```python
from build123d import *

# Parameters (mm, degrees)
F0_R     = 3.175
F0_W     = 5.842
F0_H     = 12.7
F1_DEPTH = 25.4


with BuildPart() as f1:
    # F0 (on Front) → F1 (new body)
    with BuildSketch(Plane.XZ):
        Polygon((5.842, 12.7), (5.842, 0), (66.294, 0), (66.294, 12.7), (56.134, 12.7), (56.134, 10.16), (10.16, 10.16), (10.16, 12.7), align=None)
        with BuildLine():
            ThreePointArc((-8.1826630726, -5.5069827884), (-3.1957909266, -4.5493385486), (-0.9398, 0))
            ThreePointArc((-0.9398, 0), (-4.5919612295, 5.3297205562), (-10.8806298187, 3.8475430269))
            ThreePointArc((-10.8806298187, 3.8475430269), (-12.1459778134, -1.5837270034), (-8.1826630726, -5.5069827884))
        make_face()
        with Locations((-6.6548, 0)):
            Circle(F0_R, mode=Mode.SUBTRACT)
        with BuildLine():
            Line((-0.9398, 0), (0, 0))
            Line((0, 0), (0, 12.7))
            Line((0, 12.7), (5.842, 12.7))
            Line((5.842, 12.7), (5.842, 15.24))
            Line((5.842, 15.24), (-0.508, 15.24))
            Line((-0.508, 15.24), (-10.8806298187, 3.8475430269))
            ThreePointArc((-10.8806298187, 3.8475430269), (-4.5919612295, 5.3297205562), (-0.9398, 0))
        make_face()
        with Locations((2.921, 6.35)):
            Rectangle(F0_W, F0_H)
        with BuildLine():
            Line((5.842, 0), (0, 0))
            Line((0, 0), (-0.9398, 0))
            ThreePointArc((-0.9398, 0), (-3.1957909266, -4.5493385486), (-8.1826630726, -5.5069827884))
            Line((-8.1826630726, -5.5069827884), (5.842, -9.398))
            Line((5.842, -9.398), (5.842, 0))
        make_face()
        with Locations((-6.6548, 0)):
            Circle(F0_R)
    extrude(amount=F1_DEPTH)


solid = f1.part
```
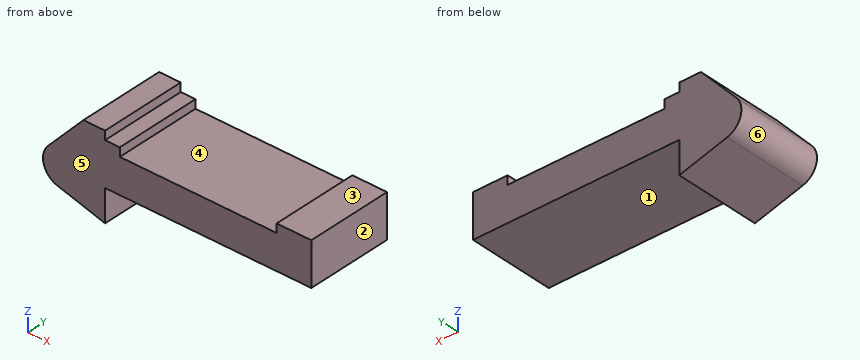
Geometry check sheet. Reference: the model listing, model coordinates, mm. Face numbers are marked on the shaded views. A direction names the side the tool comes from. Give positions to 0.01 mm unless a question says otherwise; leave off trailing zeros. Order: outer loops, then holes, each group sorted by start corner. A loop starts at its lowest first (then second) coordinate and runs counter-clockwise, first axis right, second up. Notation, with made-up numbers: (48, 89.5) -> (96, 89.5) arc R8 cw to (96, 94.5) -> close; hole circle Ø4 at (59.25, 8.5). An arc over 180 degrees is marked (long way). Write each question's results on one line, items separated by ' | '. Start each with the question number.
(1) Sectioned sample at A-A (z = 11). Enter the section's corners in (x, y).
(2) Mould release check, pull along X, two halves, no side actions. Record for the marked faces 4, 5 and 6: pulls with the +X half, pulls with the -X half, needs draft (parallel to the pull), parting line crosses it, or undercut.
(3) Access from +Z, -Z, +X, -X, +Y, -Y to the whole of each face (thin tool, end or side, straight path). Record for the marked faces 1, 2 and 3.
(4) Gauge pin test, flat ends, axial feed: P1, Ø1.3, axis at x = 8, y = -16.5, coming from the +Z side; P2, Ø4, axis at x = 40, y = -4.5, coming from the +Z side; P3, Ø5, axis at y = -19, z = 8.5, coming from the -X side. Record the tip position at first contact, or that the pin passes through.
(5) Scan lines: line 1 (Z direction, x = 19.5, y = -22.5); line 2 (X direction, y = -13, z = 11.25); line 3 (X direction, y = -7, z = 10.75). Record each from-to range of solid material in increasing order.
(6) Sectioned sample at D-D (z = -1.75). Enter the section's corners in (x, y), plus the area to 3 significant figures.
(7) Sectioned sample at C-C (x = 24). Enter the section's corners in (y, z), plus the area to 3 significant figures.
(8) Sectioned sample at B-B (y = -5). Enter the section's corners in (x, z) (3 decimals).
Answer below:
1) outline: (-4.37, -25.4) -> (10.16, -25.4) -> (10.16, 0) -> (-4.37, 0) -> close; (56.13, -25.4) -> (66.29, -25.4) -> (66.29, 0) -> (56.13, 0) -> close
2) face 4: undercut | face 5: needs draft | face 6: pulls with the -X half
3) face 1: -Z, +X, +Y, -Y | face 2: +Z, -Z, +X, +Y, -Y | face 3: +Z, +X, +Y, -Y
4) P1: z = 12.7 | P2: z = 10.16 | P3: x = -8.92
5) line 1: 0 to 10.16 | line 2: -4.14 to 10.16, 56.13 to 66.29 | line 3: -4.6 to 10.16, 56.13 to 66.29
6) outline: (-12.1, -25.4) -> (5.84, -25.4) -> (5.84, 0) -> (-12.1, 0) -> close | area: 456 mm2
7) outline: (-25.4, 0) -> (0, 0) -> (0, 10.16) -> (-25.4, 10.16) -> close | area: 258 mm2
8) outline: (-10.881, 3.848) arc R5.715 ccw to (-8.183, -5.507) -> (5.842, -9.398) -> (5.842, 0) -> (66.294, 0) -> (66.294, 12.7) -> (56.134, 12.7) -> (56.134, 10.16) -> (10.16, 10.16) -> (10.16, 12.7) -> (5.842, 12.7) -> (5.842, 15.24) -> (-0.508, 15.24) -> close
